Here's how the part is built. I have some questions about the finished solid (model axes, mm). Round coordinates to 2 decimals unless told otherwise and drop trailing zeros. Loops run counter-clockwise (first coordinate to the right, second up) from the corner with the lowest first, then second, coordinate; pieces in that order, holes last. Notation, with made-up numbers: (52.25, 42) - (74.25, 42) arc R15 ccw to (74.25, 56) - close; hole circle Ø10 at (-2.75, 79). An arc over 180 degrees is marked (long way). Answer as a JSON object with one key per item and string values. Group by question number.
1) If we mould it in two halves opening along Y, with no side actions, what happens to faces 1 (the face through (0, 0, 0)), 2 (the face through (-13.785, 6.26, -0.237))? For each: pulls with the +Y half, pulls with the -Y half, needs draft (parallel to the pull), parting line crosses it, or undercut.
2) I want a section at B-B, the plane x = -3.25. Give the number of separate pieces and of enclosed holes in the cut face, then the cut area to 3 significant figures.
3) If I drill on line 1 along Y through (x, z) = (-4.5, -0.55); line 2 along X through (y, z) = (20.25, 0); line 3 along Y through (x, z) = (-10.5, 0.15), over which ranges is the centre line in solid material (lowest first)? Write a range as [from, to].
4) Will this pin go through, and if not, where does the flat tip stop? P1, Ø4, axis at x = -6.5, y = 5, coming from the -Z side.
5) I want a section at A-A, the plane z = -0.4. Please give me the cut outline in (x, y).
from build123d import *

# Parameters (mm, degrees)
SKETCH3_R = 0.7874


with BuildPart() as part:
    # Sweep1: sweep along a path in Sketch1
    with BuildLine(Plane.XY) as sweep1_path:
        Line((0, 0), (-5.620726606, 12.053687105))
        ThreePointArc((-5.620726606, 12.053687105), (-5.766457952, 13.805447622), (-4.739872572, 15.232341099))
        ThreePointArc((-4.739872572, 15.232341099), (-7.9375, 25.684049221), (-11.135127428, 15.232341099))
        ThreePointArc((-11.135127428, 15.232341099), (-10.108542048, 13.805447622), (-10.254273394, 12.053687105))
        Line((-10.254273394, 12.053687105), (-15.875, 0))
    # Sketch3 → Sweep1 (sweep)
    with BuildSketch(Plane(origin=(0, 0, 0), x_dir=(0.9063077870366525, 0.422618261740694, 0), z_dir=(-0.422618261740694, 0.9063077870366525, 0))):
        Circle(SKETCH3_R)
    sweep(path=sweep1_path.line)


solid = part.part
Outcome:
{
 "1": {"face 1": "pulls with the -Y half", "face 2": "undercut"},
 "2": {"separate pieces": "3", "enclosed holes": "0", "area": "11.8 mm^2"},
 "3": {"line 1": "[8.32, 10.98], [14.71, 16.13], [23.81, 25.22]", "line 2": "[-14.43, -12.86], [-3.02, -1.44]", "line 3": "[9.7, 15.72], [24.19, 25.93]"},
 "4": {"P1": "through"},
 "5": {"outline": "(-16.49, 0.29) - (-15.26, -0.29) - (-9.64, 11.77) arc R3.22 ccw to (-10.76, 15.79) arc R5.04 cw (long way) to (-5.12, 15.79) arc R3.22 ccw to (-6.24, 11.77) - (-0.61, -0.29) - (0.61, 0.29) - (-5.01, 12.34) arc R1.86 cw to (-4.36, 14.67) arc R6.39 ccw (long way) to (-11.51, 14.67) arc R1.86 cw to (-10.87, 12.34) - close"}
}
